Verification items for the finished model (mm, model axes). Coordinates: 2 decimals unless noted, no trailing zeros. Write each loop counter-clockwise with the first axis right and the second up, starting at its lowest first coordinate (ties: lowest second). Pieces come first, ordered by that corner, then holes. Notation, with made-up numbers: (-37.75, 61) -> (6.25, 61) arc R17 ccw to (6.25, 74) -> close; hole circle Ø3 at (2, -24.5). An arc over 180 degrees is marked (long way). Write item = value, one per line. Start each with the question number.
(1) Section check C-C (y = 107). Record the cut outline in (x, z), plus the area to 3 significant figures.
(2) Material ranges on probe 1 along Y at (x, z) = (7, 0); probe 2 along Y at (x, z) = (4, -1); probe 3 along X at (y, z) = (55, 0.25), recorded low to high. Write a range as [from, to].
(3) Section check A-A (z = 0). Record the cut outline in (x, y).
(4) Section check B-B (x = 4.5). Record the cut outline in (y, z) (3 decimals), plus the area to 3 significant figures.
(5) Gauge pin test, flat ends, axial feed: pin 1 Ø4 at (y, z) = (230.5, 2.5) entering from -X; pin 2 Ø7 at (y, z) = (498, 1.5) entering from +X; pin 3 Ø1.9 at (y, z) = (9.5, 1) entering from +X; pin 4 Ø8 at (y, z) = (84, 6.5) entering from -X. Record the tip position at first contact, or that the pin passes through.
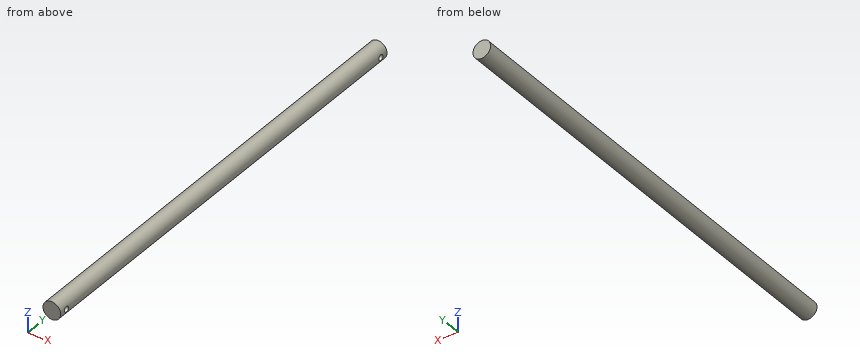
```python
from build123d import *

# Parameters (mm, degrees)
SKETCH1_R           = 9.906
BOSS_EXTRUDE1_DEPTH = 508
CUT_EXTRUDE1_START  = 20.32
SKETCH2_R           = 3.175
CUT_EXTRUDE1_DEPTH  = 22.86


with BuildPart() as part:
    # Sketch1 → Boss-Extrude1 (new body)
    with BuildSketch(Plane(origin=(0, 0, 0), x_dir=(1, 0, 0), z_dir=(0, 1, 0))):
        with Locations(Location((0, 0, 0), (0, 0, 270))):
            Circle(SKETCH1_R)
    extrude(amount=BOSS_EXTRUDE1_DEPTH)

    # Sketch2 → Cut-Extrude1 (cut)
    with BuildSketch(Plane(origin=(0, 0, 0), x_dir=(0, 0, -1), z_dir=(1, 0, 0)).offset(CUT_EXTRUDE1_START)):
        with Locations((0, 498.602)):
            Circle(SKETCH2_R)
    cut_extrude1 = extrude(amount=-CUT_EXTRUDE1_DEPTH, mode=Mode.SUBTRACT)

    # Mirror1: Cut-Extrude1 across plane
    add(cut_extrude1.mirror(Plane.ZX.offset(254)), mode=Mode.SUBTRACT)


solid = part.part
```
Response:
q1.outline = circle Ø19.81 at (0, 0)
q1.area = 308 mm2
q2.probe_1 = [0, 6.22], [12.57, 495.43], [501.78, 508]
q2.probe_2 = [0, 6.38], [12.41, 495.59], [501.62, 508]
q2.probe_3 = [-9.9, 9.9]
q3.outline = (-9.91, 0) -> (9.91, 0) -> (9.91, 6.22) -> (-2.54, 6.22) -> (-2.54, 12.57) -> (9.91, 12.57) -> (9.91, 495.43) -> (-2.54, 495.43) -> (-2.54, 501.78) -> (9.91, 501.78) -> (9.91, 508) -> (-9.91, 508) -> close
q4.outline = (0, -8.825) -> (508, -8.825) -> (508, 8.825) -> (0, 8.825) -> close; hole circle Ø6.35 at (9.398, 0); hole circle Ø6.35 at (498.602, 0)
q4.area = 8,900 mm2
q5.pin_1 = -9.89
q5.pin_2 = 9.91
q5.pin_3 = -2.54
q5.pin_4 = -9.59
